```python
from build123d import *

# Parameters (mm, degrees)
BOSS_EXTRUDE1_DEPTH = 6
FILLET1_R           = 0.5
SKETCH4_R           = 6
BOSS_EXTRUDE2_DEPTH = 6
SKETCH3_R           = 6
SKETCH3_R_2         = 2
CUT_EXTRUDE1_DEPTH  = 377.172507901


with BuildPart() as part:
    # Sketch2 → Boss-Extrude1 (new body)
    with BuildSketch(Plane(origin=(0, 0, 0), x_dir=(0, 0, -1), z_dir=(1, 0, 0))):
        Polygon((0, 376), (0, 0), (-25, 25), (-25, 351), align=None)
    extrude(amount=BOSS_EXTRUDE1_DEPTH)

    # Fillet1
    fillet1_edges = [part.edges().sort_by_distance(p)[0] for p in [
        (3, 376, 0),
        (3, 0, 0),
    ]]
    fillet(fillet1_edges, radius=FILLET1_R)

    # Sketch4 → Boss-Extrude2 (add)
    with BuildSketch(Plane.ZY):
        with Locations((12, 12)):
            Circle(SKETCH4_R)
    extrude(amount=-BOSS_EXTRUDE2_DEPTH)

    # Sketch3 → Cut-Extrude1 (cut, through all)
    with BuildSketch(Plane(origin=(6, 0, 0), x_dir=(0, 0, -1), z_dir=(1, 0, 0))):
        with Locations((-12, 364)):
            Circle(SKETCH3_R)
        with Locations((-12, 12)):
            Circle(SKETCH3_R_2)
    extrude(amount=-CUT_EXTRUDE1_DEPTH, mode=Mode.SUBTRACT)


solid = part.part
```
Input: part model. Units: mm. Frame: model coordinates. A direction names the side the tool comes from. Give positions to 0.01 mm unless a question says otherwise; leave off trailing zeros. Write each loop counter-clockwise with the first axis right and the second up, starting at its lowest first coordinate (ties: lowest second). Pieces come first, ordered by that corner, then holes. Notation, with made-up numbers: (64.5, 27) - (89.5, 27) arc R29 ccw to (89.5, 56) - close; hole circle Ø3 at (-9, 77). An arc over 180 degrees is marked (long way). Write item = value, one per line. Start each with the question number.
1) Cut plane A-A (x = 4.95). Return loops of the section in (y, z).
2) Draft query along Y for faces 1 (the face through (3.042, 359.665, 7.852)), 2 (the face through (0, 191, 12)), 3 (the face through (3, 4, 4)). Return one class per face: pulls with the +Y half, pulls with the -Y half, needs draft (parallel to the pull), parting line crosses it, or undercut.
3) Reachability of faces 4 (the face through (3, 21, 21)), 5 (the face through (3, 372, 4)) from +Z, -Z, +X, -X, +Y, -Y: full face, straight path, thin tool, end or side. Return the list, or none.
4) Pin query (flat end, axial travel): pin 1 (2.5 mm diameter, centred on y = 12, z = 12, fed in from +X); pin 2 (1.5 mm diameter, centred on x = 5.5, z = 8.5, fed in from -Y). Return the tip coordinate at first contact, or that it passes through.
5) Cut plane B-B (y = 364). Return loops of the section in (x, z).
6) Material intervals for L1, parallel to Y at x = 2.9, z = 12; L2, parallel to Y at x = 0.8, z = 23; L3, parallel to Y at x = 4.9, z = 18.75, sorted ascending. Write a range as [from, to].
Answers follow:
q1.outline = (0.85, 0.85) arc R0.5 ccw to (1.21, 0) - (374.79, 0) arc R0.5 ccw to (375.15, 0.85) - (368.24, 7.76) arc R6 cw to (359.76, 16.24) - (351, 25) - (25, 25) - (16.24, 16.24) arc R6 ccw to (7.76, 7.76) - close; hole circle Ø4 at (12, 12)
q2.face_1 = undercut
q2.face_2 = needs draft
q2.face_3 = pulls with the -Y half
q3.face_4 = +Z, +X, -X
q3.face_5 = +Z, +X, -X, +Y
q4.pin_1 = through
q4.pin_2 = 6.67
q5.outline = (0, 0) - (6, 0) - (6, 6) - (0, 6) - close
q6.L1 = [6, 10], [14, 358]
q6.L2 = [23, 353]
q6.L3 = [18.75, 357.25]
